from build123d import *

# Parameters (mm, degrees)
SKETCH1_W           = 60
SKETCH1_H           = 30
BOSS_EXTRUDE1_DEPTH = 5
SKETCH2_W           = 60
SKETCH2_H           = 15
BOSS_EXTRUDE2_DEPTH = 70
SKETCH3_R           = 20
CUT_EXTRUDE1_DEPTH  = 10
SKETCH4_R           = 2.5
CUT_EXTRUDE2_DEPTH  = 5
FILLET1_R           = 30


with BuildPart() as part:
    # Sketch1 → Boss-Extrude1 (new body)
    with BuildSketch(Plane.XY):
        Rectangle(SKETCH1_W, SKETCH1_H)
    extrude(amount=BOSS_EXTRUDE1_DEPTH)

    # Sketch2 → Boss-Extrude2 (add)
    with BuildSketch(Plane.XY.offset(5)):
        with Locations((0, -7.5)):
            Rectangle(SKETCH2_W, SKETCH2_H)
    extrude(amount=BOSS_EXTRUDE2_DEPTH)

    # Sketch3 → Cut-Extrude1 (cut)
    with BuildSketch(Plane(origin=(0, 0, 0), x_dir=(1, 0, 0), z_dir=(0, 1, 0))):
        with Locations(Location((0, -50, 0), (0, 0, 270))):
            Circle(SKETCH3_R)
    extrude(amount=-CUT_EXTRUDE1_DEPTH, mode=Mode.SUBTRACT)

    # Sketch4 → Cut-Extrude2 (cut)
    with BuildSketch(Plane(origin=(0, 0, 0), x_dir=(-1, 0, 0), z_dir=(0, 0, -1))):
        with Locations((-17.5, 10)):
            Circle(SKETCH4_R)
        with Locations((17.5, 10)):
            Circle(SKETCH4_R)
        with Locations((17.5, -5)):
            Circle(SKETCH4_R)
        with Locations((-17.5, -5)):
            Circle(SKETCH4_R)
    extrude(amount=-CUT_EXTRUDE2_DEPTH, mode=Mode.SUBTRACT)

    # Fillet1
    fillet1_edges = [part.edges().sort_by_distance(p)[0] for p in [
        (30, -7.5, 75),
        (-30, -7.5, 75),
    ]]
    fillet(fillet1_edges, radius=FILLET1_R - 0.0001)  # a hair under: the kernel refuses the full size


solid = part.part
Geometry: final body of the model. Coordinates: model frame, mm. A direction names the side the tool comes from. Give positions to 0.01 mm unless a question says otherwise; leave off trailing zeros. Order: outer loops, then holes, each group sorted by start corner. A loop starts at its lowest first (then second) coordinate and runs counter-clockwise, first axis right, second up. Notation, with made-up numbers: (44.25, -22.5) -> (80.25, -22.5) arc R17 ccw to (80.25, 10.5) -> close; hole circle Ø10 at (75.5, 80). An arc over 180 degrees is marked (long way). Put each result on its own line as item: value.
Q1. Material intervals for L1, parallel to Y at x = 17.5, z = 2.35; L2, parallel to Y at x = 17, z = 3; L3, parallel to Y at x = 4.5, z = 33, sorted ascending.
Here are the results:
L1: y = -15 to -7.5, -2.5 to 7.5, 12.5 to 15
L2: y = -15 to -7.45, -2.55 to 7.55, 12.45 to 15
L3: y = -15 to -10
Q2. Pin query (flat end, axial travel): pin 1 (6 mm diameter, centred on x = 17, z = 45.5, fed in from +Y); pin 2 (4.5 mm diameter, centred on x = -17.5, y = -5, fed in from -Z); pin 3 (6 mm diameter, centred on y = 5.5, z = 35, fed in from -X); pin 4 (8 mm diameter, centred on x = 17.5, y = -5, fed in from +Z). Return the tip coordinate at first contact, or that it passes through.
Here are the results:
pin 1: stops at y = 0
pin 2: stops at z = 5
pin 3: passes through
pin 4: stops at z = 71.79
Q3. Reachability of faces 5 (the face through (6.007, -4.93, 69.076)), 6 (the face through (-15, -5, 2)), 7 (the face through (0, 8, 5)), 8 (the face through (20.979, -7.395, 66.445)) from +Z, -Z, +X, -X, +Y, -Y: full face, straight path, thin tool, end or side. Return the list, or none.
Here are the results:
face 5: +Y
face 6: -Z
face 7: +Z, +X, -X, +Y
face 8: +Z, +X, +Y, -Y
Q4. Section C-C, the plane x = -17.5. Return loops of the section in (y, z), then the cut area to 3 significant figures.
Here are the results:
outline: (-15, 0) -> (-7.5, 0) -> (-7.5, 5) -> (-2.5, 5) -> (-2.5, 0) -> (7.5, 0) -> (7.5, 5) -> (0, 5) -> (0, 40.32) -> (-10, 40.32) -> (-10, 59.68) -> (0, 59.68) -> (0, 69.37) -> (-15, 69.37) -> close; (12.5, 0) -> (15, 0) -> (15, 5) -> (12.5, 5) -> close
area: 872 mm^2
Q5. Draft query along Y for faces 1 (the face through (-21.445, -7.395, 65.979)), 2 (the face through (20, -5, 2)), 3 (the face through (0, -15, 37)), 4 (the face through (-16, 8, 2)). Return one class per face: released by +Y, released by -Y, zero draft, split by the parting line, or undercut.
Here are the results:
face 1: zero draft
face 2: undercut
face 3: released by -Y
face 4: undercut
Q6. Section A-A, the plane y = 10. Return loops of the section in (x, z), then the cut area to 3 significant figures.
Here are the results:
outline: (-30, 0) -> (-20, 0) -> (-20, 5) -> (-30, 5) -> close; (-15, 0) -> (15, 0) -> (15, 5) -> (-15, 5) -> close; (20, 0) -> (30, 0) -> (30, 5) -> (20, 5) -> close
area: 250 mm^2
Q7. Section D-D, the plane z = 60.5. Return loops of the section in (x, y).
Here are the results:
outline: (-25.69, -15) -> (25.69, -15) -> (25.69, 0) -> (17.02, 0) -> (17.02, -10) -> (-17.02, -10) -> (-17.02, 0) -> (-25.69, 0) -> close
